Design review of the part built by this model. Coordinates are the model's own, in mm. Face numbers are marked on the shaded views. A direction names the side the tool comes from. Round coordinates to 2 decimals unless told otherwise and drop trailing zeros. Order: outer loops, then holes, each group sorted by start corner. A loop starts at its lowest first (then second) coordinate and runs counter-clockwise, first axis right, second up. Notation, with made-up numbers: (-2.5, 73.25) - (6.5, 73.25) arc R21 ccw to (6.5, 107.25) - close; hole circle Ø2 at (14, 26.25). An arc over 180 degrees is marked (long way). Write item = value, one per line.
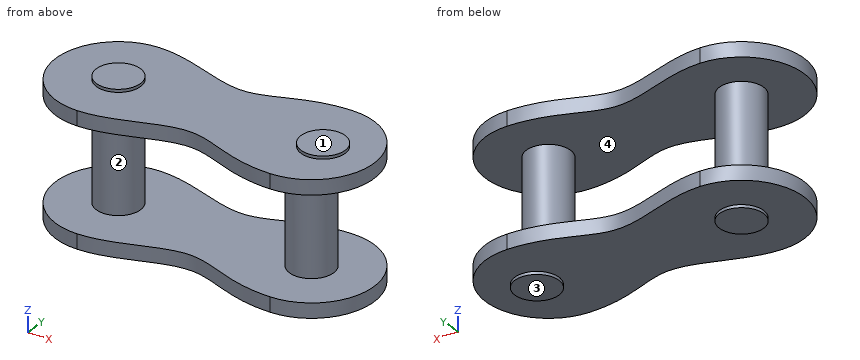
from build123d import *

# Parameters (mm, degrees)
SKETCH1_R               = 1.5
BOSS_EXTRUDE6_DEPTH     = 9
BOSS_EXTRUDE6_2_DEPTH   = 9
BOSS_EXTRUDE7_DEPTH     = 1
SKETCH6_R               = 1.5
BOSS_EXTRUDE8_DEPTH     = 0.2
CUT_EXTRUDE1_DEPTH      = 21.485726843
CUT_EXTRUDE1_DEPTH_BACK = 21.485726843


with BuildPart() as part:
    # Sketch1 → Boss-Extrude6 (new body)
    with BuildSketch(Plane.XY):
        Circle(SKETCH1_R)
    extrude(amount=BOSS_EXTRUDE6_DEPTH)



with BuildPart() as body_2:
    # Sketch1 → Boss-Extrude6 2 (new body)
    with BuildSketch(Plane.XY):
        with Locations((13, 0)):
            Circle(SKETCH1_R)
    extrude(amount=BOSS_EXTRUDE6_2_DEPTH)


with BuildPart() as part_1:
    add(part.part)

    add(body_2.part)  # Boss-Extrude7 merges body 2
    # Sketch5 → Boss-Extrude7 (add)
    with BuildSketch(Plane.XY.offset(9)):
        with BuildLine():
            ThreePointArc((0, 4.25), (-4.25, 0), (0, -4.25))
            add(Edge.make_bspline(
                [(0, -4.25), (2.386303511, -4.25), (6.863643386, -1.25), (9.886409718, -4.25), (13, -4.25)],
                knots=[0, 0, 0, 0, 0.5, 1, 1, 1, 1], degree=3))
            ThreePointArc((13, -4.25), (17.25, 0), (13, 4.25))
            add(Edge.make_bspline(
                [(0, 4.25), (2.386303511, 4.25), (6.863643386, 1.25), (9.886409718, 4.25), (13, 4.25)],
                knots=[0, 0, 0, 0, 0.5, 1, 1, 1, 1], degree=3))
        make_face()
    boss_extrude7 = extrude(amount=BOSS_EXTRUDE7_DEPTH)

    # Sketch6 → Boss-Extrude8 (add)
    with BuildSketch(Plane.XY.offset(10)):
        Circle(SKETCH6_R)
        with Locations((13.777718246, 0)):
            Circle(SKETCH6_R)
    boss_extrude8 = extrude(amount=BOSS_EXTRUDE8_DEPTH)

    # Sketch8 → Cut-Extrude1 (cut, two sides: drawn at the far end of the back side and taken through both)
    with BuildSketch(Plane(origin=(0, 0, 0), x_dir=(0, 0, -1), z_dir=(1, 0, 0)).offset(-CUT_EXTRUDE1_DEPTH_BACK)):
        Polygon((0, 0), (0, 2.418260543), (-2, 2.418260543), (-2, -2.301811822), (0, -2.301811822), align=None)
    extrude(amount=CUT_EXTRUDE1_DEPTH + CUT_EXTRUDE1_DEPTH_BACK, mode=Mode.SUBTRACT)

    # Mirror1: Boss-Extrude7, Boss-Extrude8 across plane
    add(boss_extrude7.mirror(Plane(origin=(0, 0, 5.5), x_dir=(1, 0, 0), z_dir=(0, 0, -1))))
    add(boss_extrude8.mirror(Plane(origin=(0, 0, 5.5), x_dir=(1, 0, 0), z_dir=(0, 0, -1))))


solid = part_1.part
1) Clearance check with flat-ended pins moving along their axes: pin 1 Ø4.5 at (x, y) = (8, 1) entering from +Z; pin 2 Ø1.5 at (y, z) = (-2, 3.5) entering from +X; pin 3 Ø1.5 at (x, z) = (6, 7.5) entering from -Y. State where each tip first meets the part, or that it passes through.
Findings:
pin_1 = 10
pin_2 = 13.83
pin_3 = through
2) The part is to be moulded in two halves that separate along X. For the marked faces 3 and 4, say which applies: released by +X, released by -X, zero draft, split by the parting line, or undercut.
Findings:
face_3 = zero draft
face_4 = undercut
3) We need section C-C on x = -1. Write out the cut boundary in (y, z).
Findings:
outline = (-4.13, 1) - (-1.12, 1) - (-1.12, 0.8) - (1.12, 0.8) - (1.12, 1) - (4.13, 1) - (4.13, 2) - (1.12, 2) - (1.12, 9) - (4.13, 9) - (4.13, 10) - (1.12, 10) - (1.12, 10.2) - (-1.12, 10.2) - (-1.12, 10) - (-4.13, 10) - (-4.13, 9) - (-1.12, 9) - (-1.12, 2) - (-4.13, 2) - close
4) We need section B-B on z = 2.5. Write out the cut boundary in (x, y).
Findings:
outline = circle Ø3 at (0, 0); circle Ø3 at (13, 0)
5) To check wall thickness, follow L1, parallel to Z at x = 7, y = 1; L2, parallel to X at y = 0.5, z = 7.75; L3, parallel to X at y = -0.25, z = 4.25. State the ranges of each line that lie inside material, in increasing order. Write a range as from..to.
Findings:
L1 = 1..2, 9..10
L2 = -1.41..1.41, 11.59..14.41
L3 = -1.48..1.48, 11.52..14.48
6) For the marked faces 1 and 2, list the 3-axis set-ups (+Z, -Z, +X, -X, +Y, -Y) from which the entire face can be reached by the end or side of a thin tool; tool diameter is ignored.
Findings:
face_1 = +Z, +X, -X, +Y, -Y
face_2 = none
